Autodesk Fusion 360 part; units mm, degrees
sketch "bottom" plane through (0, 0, 0) normal (0, 0, 1) x (1, 0, 0)
  circle A0 centre (0, 0) radius 2.25
  line L0 (4.15, 0) -> (2.075, 3.594)
  line L1 (2.075, 3.594) -> (-2.075, 3.594)
  line L2 (-2.075, 3.594) -> (-4.15, 0)
  line L3 (-4.15, 0) -> (-2.075, -3.594)
  line L4 (-2.075, -3.594) -> (2.075, -3.594)
  line L5 (2.075, -3.594) -> (4.15, 0)
  line L6 (4.75, 6.25) -> (-4.75, 6.25)
  line L7 (-6.25, 4.75) -> (-6.25, -4.75)
  line L8 (-4.75, -6.25) -> (4.75, -6.25)
  line L9 (6.25, -4.75) -> (6.25, 4.75)
  line L10 (6.25, 6.25) -> (-6.25, -6.25) construction
  line L11 (-6.25, 6.25) -> (6.25, -6.25) construction
  arc A1 (4.75, -6.25) -> (6.25, -4.75) centre (4.75, -4.75) ccw
  arc A2 (-6.25, -4.75) -> (-4.75, -6.25) centre (-4.75, -4.75) ccw
  arc A3 (-4.75, 6.25) -> (-6.25, 4.75) centre (-4.75, 4.75) ccw
  arc A4 (6.25, 4.75) -> (4.75, 6.25) centre (4.75, 4.75) ccw
  circle A5 centre (0, 0) radius 20
  circle A6 centre (0, 0) radius 55
  line L12 (0, 55) -> (0, 52)
  line L13 (0, 55) -> (10.5968, 49.8773)
  line L14 (0, 55) -> (11.77, 55) construction
  line L15 (0, 52) -> (10.5968, 46.8773)
  arc A7 (25.1153, 10.0637) -> (9.1347, 47.5841) centre (-4.3574, 19.6742) ccw
  arc A8 (19.7662, -3.0491) -> (10.5968, 49.8773) centre (-2.8509, 20.29) ccw
  spline S0 degree 5 poles (19.2844, 5.302) (19.288, 5.2968) (19.3924, 5.1455) (19.6116, 4.8896) (19.9793, 4.632) (20.5483, 4.5429) (21.3688, 4.8461) (22.2615, 5.515) (23.1597, 6.4634) (23.9893, 7.5946) (24.5403, 8.5729) (24.8652, 9.3175) (25.039, 9.8148) (25.1153, 10.0637) knots 0.196493 0.196493 0.196493 0.196493 0.196493 0.196493 0.2 0.3 0.4 0.5 0.6 0.7 0.8 0.9 1 1 1 1 1 1
  line L16 (18.6573, 6.2172) -> (19.9116, 4.3867)
  line L17 (24.8256, 9.1182) -> (25.4049, 11.0092)
  point P0 (20.8497, 4.7036)
  dimension "d1" = 4.5
  dimension "d2" = 4.15
  dimension "d3" = 12.5
  dimension "d4" = 12.5
  dimension "d5" = 1.5
  dimension "d6" = 1.5
  dimension "d7" = 1.5
  dimension "d8" = 40
  dimension "d9" = 110
  dimension "d10" = 3
  dimension "d11" = 25.8
  dimension "d12" = 11.77
  dimension "d13" = 11.77
  dimension "d14" = 62
  dimension "d16" = 65
extrude "Extrude2" add sketch "bottom" along normal blind 8 contours A5 L12 L13 L15 A7 A8 S0 L17 makes body 1
pattern_circular "C-Pattern1" count 5 over 360 about axis through (0, 0, 0) along (0, 0, 1) of "Extrude2" makes body 2 makes body 3 makes body 4 makes body 5
extrude "Extrude3" add sketch "bottom" along normal blind 8 contours L0 L1 L2 L3 L4 L5 | L6 L7 L8 L9 A1 A2 A3 A4 | A5 bodies 1 2 3 4 5
extrude "Extrude4" add sketch "bottom" along normal blind 31.5 contours L0 L1 L2 L3 L4 L5 | L6 L7 L8 L9 A1 A2 A3 A4 bodies 1
extrude "Extrude5" cut sketch "bottom" along normal blind 4 contours L0 L1 L2 L3 L4 L5 bodies 1
equation "d2 = ( 8.3 / 2 ) * 1 mm"
equation "d11 = 90 deg - 64.2 deg"
Work out the finished part from the listing and answer in its coordinate system (mm). A direction names the side the tool comes from. Coordinates: 2 decimals unless noted, no trailing zeros. Loops run counter-clockwise (first coordinate to the right, second up) from the corner with the lowest first, then second, coordinate; pieces in that order, holes last. Notation, with made-up numbers: (3.5, 27.25) - (37.5, 27.25) arc R26 ccw to (37.5, 44.25) - close; hole circle Ø7 at (60.5, 23). An arc over 180 degrees is marked (long way). Use a Markdown table: item, result.
Item 1: Given pin 1 Ø7.5 at (y, z) = (0, 21.5) entering from +X; pin 2 Ø7.5 at (x, z) = (-1, 25) entering from -Y; pin 3 Ø8 at (x, y) = (1, -1) entering from -Z; pin 4 Ø1.2 at (x, z) = (0.5, 2) entering from -Y, each flat-ended and moving along its own axis, determine where each tip first touches the part or whether it passes through.
Evaluation:
| item | result |
|---|---|
| pin 1 | stops at x = 6.25 |
| pin 2 | stops at y = -6.25 |
| pin 3 | stops at z = 0 |
| pin 4 | stops at y = -44.47 |
Item 2: Find section A-A, the plane z = 21.5. Determine the outline of the cut face in (x, y), and give its area (3 significant figures).
Evaluation:
| item | result |
|---|---|
| outline | (-6.25, -4.75) arc R1.5 ccw to (-4.75, -6.25) - (4.75, -6.25) arc R1.5 ccw to (6.25, -4.75) - (6.25, 4.75) arc R1.5 ccw to (4.75, 6.25) - (-4.75, 6.25) arc R1.5 ccw to (-6.25, 4.75) - close; hole circle Ø4.5 at (0, 0) |
| area | 138 mm2 |
Item 3: The mould has two halves that part along Y. Classify faces 1 (the flat face through (5.224, 52.475, 3.944)), 2 (the flat face through (-32.93, -37.66, 3.94)), 3 (the flat face through (-45.99, 19.68, 3.94)): +Y half, -Y half, draft (parallel to the pull), parting line (faces both ways), or undercut.
Evaluation:
| item | result |
|---|---|
| face 1 | +Y half |
| face 2 | undercut |
| face 3 | -Y half |
Item 4: Consider probe 1 along Y at (x, z) = (0, 11); probe 2 along Z at (x, y) = (-24.5, 10); probe 3 along X at (y, z) = (-26, 2.5). Determine where each line is inside the solid, lowest interval first. Write a range as from..to.
Evaluation:
| item | result |
|---|---|
| probe 1 | y = -6.25..-2.25, 2.25..6.25 |
| probe 2 | z = 0..8 |
| probe 3 | x = -41.14..-38.11, -16.25..-13.21 |
Item 5: For faces 4 (the flat face through (50.9, 16.54, 3.94)), 5 (the cylindrical face through (-7.374, 18.591, 3.944)), 6 (the flat face through (3.13, 1.77, 1.97)), 7 (the flat face through (6.25, 0, 20)), determine the directions among +Z, -Z, +X, -X, +Y, -Y from which every point of the face is accessible in a straight line to the end or side of a thin tool.
Evaluation:
| item | result |
|---|---|
| face 4 | +Z, -Z, +Y |
| face 5 | +Z, -Z |
| face 6 | -Z |
| face 7 | +Z, +X, +Y, -Y |
